Could you check a few things on this drawing? It's one solid part, dimensions in mm from its lowest x, y, z. Coordinates: 2 decimals unless noted, no trailing zeros. Order: outer loops, then holes, each group sorted by start corner. A loop starts at its lowest first (then second) coordinate and runs counter-clockwise, first axis right, second up. Notation, with made-up numbers: (51, 26) -> (64, 26) arc R26 ccw to (64, 60) -> close; hole circle Ø6 at (-36, 68). An arc over 180 degrees is marked (long way). Answer as CSV lines item,"result".
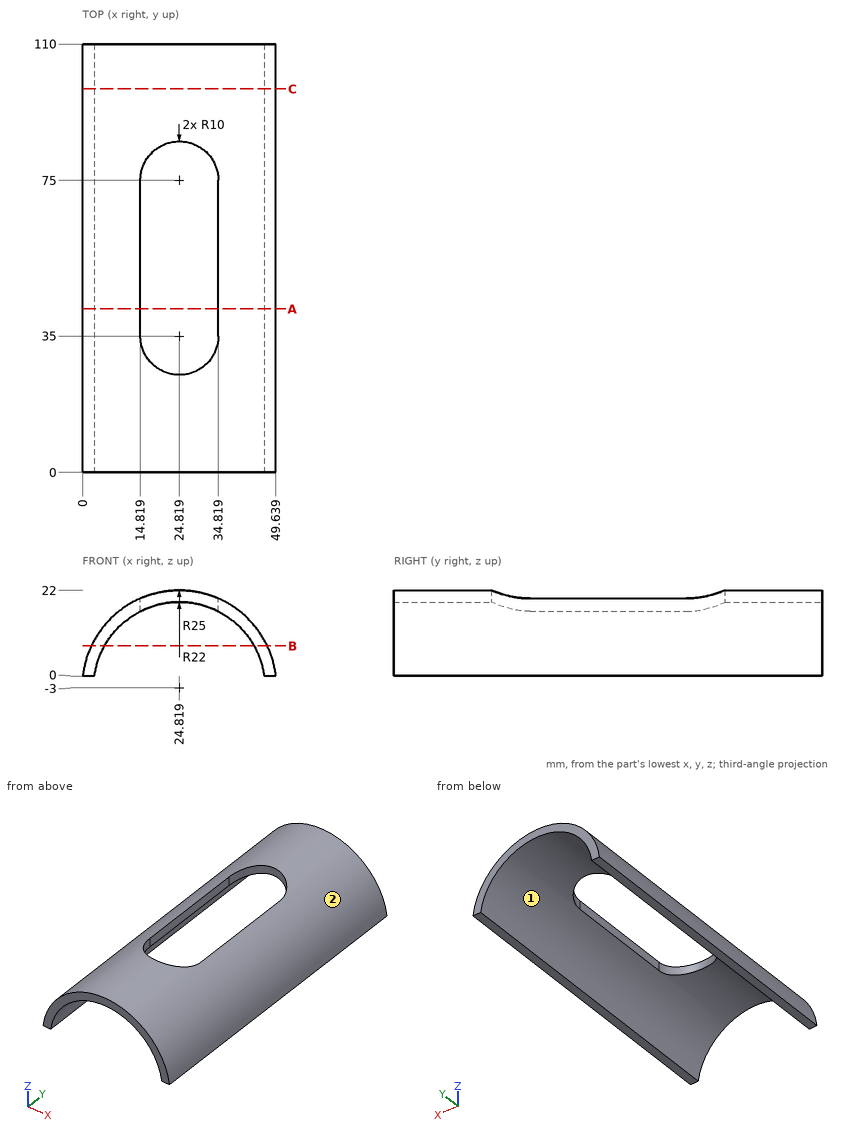
Q1. If I drill on line 1 (X direction, y = 40, z = 19.5) (1 decimal); line 2 (X direction, y = 79, z = 11); line 3 (Z direction, x = 13.5, y = 48.5) (1 decimal), over which ranges is the centre line in solid material (lowest first)?
Solution:
line 1,"13.9 to 14.8, 34.8 to 35.7"
line 2,"4.11 to 7.85, 41.79 to 45.53"
line 3,"15.9 to 19.3"
Q2. For P1, Ø4, axis at y = 98, z = 18.5, coming from the -X side (1 decimal); P2, Ø1.7, axis at y = 53.5, z = 17.5, coming from the +X side (1 decimal); P3, Ø3, axis at x = 33.5, y = 63, coming from the +Z side; P4, Ø2, axis at x = 22.5, y = 83, coming from the -Z side, each with a flat end and sliding along its axis, tell me the tip position at first contact or that it passes through.
Solution:
P1,"x = 9.2"
P2,"x = 40.3"
P3,"z = 19.91"
P4,"through"
Q3. Imagine slicing it at C-C (y = 98.5). List the corners of the cut face in (x, z) for me (1 decimal).
Solution:
outline,"(0, 0) -> (3, 0) arc R22 cw to (46.6, 0) -> (49.6, 0) arc R25 ccw to start"
Q4. Imagine slicing it at B-B (z = 7.75). List the corners of the cut face in (x, y) for me (1 decimal).
Solution:
outline,"(2.2, 0) -> (5.6, 0) -> (5.6, 110) -> (2.2, 110) -> close; (44, 0) -> (47.4, 0) -> (47.4, 110) -> (44, 110) -> close"
Q5. We'd pull the mould along X, two halves only. Please class the marked faces 1 and 2: pulls with the +X half, pulls with the -X half, needs draft (parallel to the pull), parting line crosses it, or undercut.
Solution:
face 1,"undercut"
face 2,"parting line crosses it"
Q6. Imagine slicing it at A-A (y = 42). List the corners of the cut face in (x, z) for me (1 decimal).
Solution:
outline,"(0, 0) -> (3, 0) arc R22 cw to (14.8, 16.6) -> (14.8, 19.9) arc R25 ccw to start; (34.8, 16.6) arc R22 cw to (46.6, 0) -> (49.6, 0) arc R25 ccw to (34.8, 19.9) -> close"
